Check sheet for the modelled part. Datum: model origin and axes. Units: mm. A direction names the side the tool comes from. Coordinates: 2 decimals unless noted, no trailing zeros. Write each loop counter-clockwise with the first axis right and the second up, starting at its lowest first coordinate (ties: lowest second). Pieces come first, ordered by that corner, then holes. Notation, with made-up numbers: (82, 46.5) - (131, 46.5) arc R24 cw to (131, 72.5) - close; hole circle Ø4 at (61.25, 86). An arc over 180 degrees is marked (long way). Use one line per item in the form item = value. Start each with the question number.
1. Cross-section at B-B on y = 36.5. Record the boundary of the cut face in (x, z).
2. Cross-section at A-A on z = 5.25. Give the number of separate pieces and of enclosed holes in the cut face, then the cut area to 3 significant figures.
3. Scan lines: line 1 along Y through (x, z) = (9.5, 5.5); line 2 along Z through (x, y) = (-29, 30); line 3 along Y through (x, z) = (0, 6.75). Record each from-to range of solid material in increasing order.
4. Draft check along X on faces 1 (the face through (-33.92, 88.5, 6.9)), 2 (the face through (31, 45, 9)), 3 (the face through (-19, 45, 9)), 4 (the face through (13, 55, 14)). Enter one of: +X half, -X half, draft (parallel to the pull), parting line (faces both ways), or undercut.
5. Go/stop test with flat-tipped pins: pin 1 Ø3 at (y, z) = (7.5, 9.5) entering from -X; pin 2 Ø24 at (x, y) = (1, 66) entering from -Z; pin 3 Ø2 at (x, z) = (52.5, 4.5) entering from +Y; pin 4 Ø4 at (x, z) = (42, 11.5) entering from +Y. Record where each tip stops, or that it passes through.
6. Tool access check on faces 5 (the face through (27.92, 47.55, 4.44)), 6 (the face through (6.2, 15, 6.9)), 7 (the face through (59.499, 37, 7)). Record the directions out of +Z, -Z, +X, -X, +Y, -Y that give a thin tool (end or side, any length) a straight path to the whole face; none if there is none.
Autodesk Inventor part; units mm, degrees
ref_plane "YZ Plane" through (0, 0, 0) normal (1, 0, 0) x (0, 1, 0)
ref_plane "XZ Plane" through (0, 0, 0) normal (0, 1, 0) x (-1, 0, 0)
ref_plane "XY Plane" through (0, 0, 0) normal (0, 0, 1) x (1, 0, 0)
sketch "Sketch1" plane through (0, 0, 0) normal (0, 0, 1) x (1, 0, 0)
  line L0 (11.0906, 0.1113) -> (11.0906, 10.1113)
  line L1 (11.0906, 10.1113) -> (1.0906, 20.1113)
  line L2 (31.0918, 20.1126) -> (21.0906, 10.1113)
  line L3 (21.0906, 10.1113) -> (21.0906, 0.1113)
  line L4 (21.0906, 0.1113) -> (11.0906, 0.1113)
  circle A0 centre (16.0906, 16.0413) radius 3.9
  line L5 (37.1863, 89.9817) -> (4.7287, 98.6787)
  line L6 (41.216, 88.9019) -> (37.1863, 89.9817)
  circle A1 centre (31.0906, 45.1113) radius 4
  circle A2 centre (-18.9094, 45.1113) radius 4
  line L7 (1.0906, 20.1113) -> (-38.9094, 20.1113)
  line L8 (4.7287, 98.6787) -> (-28.7852, 107.6587)
  circle A3 centre (6.0906, 62.1113) radius 9
  line L9 (-38.9094, 69.8746) -> (-28.7852, 107.6587)
  line L10 (31.0918, 20.1126) -> (59.4992, 20.1126)
  line L11 (59.4992, 20.1126) -> (59.4992, 54.8735)
  line L12 (59.4992, 84.003) -> (41.216, 88.9019)
  line L13 (59.4992, 54.8735) -> (66.7815, 82.0517)
  line L14 (66.7815, 82.0517) -> (59.4992, 84.003)
  circle A4 centre (48.4066, 52.1126) radius 3.9
  line L15 (-38.9094, 69.8746) -> (-38.9094, 20.1113)
  point P0 (0, 0)
  dimension "d2" = 10
  dimension "d5" = 135
  dimension "d6" = 135
  dimension "d7" = 10
  dimension "d8" = 10
  dimension "d11" = 7.8
  dimension "d14" = 8
  dimension "d15" = 8
  dimension "d16" = 50
  dimension "d20" = 18
  dimension "d21" = 17
  dimension "d24" = 25
  dimension "d30" = 90
  dimension "d31" = 39.117
  dimension "d51" = 7.8
  dimension "d52" = 10
  dimension "d53" = 32
  dimension "d71" = 34.7609
  dimension "d72" = 25
  dimension "d73" = 25
  dimension "d74" = 5
  dimension "d75" = 49.7632
  dimension "d77" = 28.4086
extrude "Extrusion6" add sketch "Sketch1" along normal blind 14
sketch "Sketch6" plane through (59.4992, 20.1126, 0) normal (1, 0, 0) x (0, 0, -1)
  circle A0 centre (-7, 10.2998) radius 3.8217
  line L0 (0, -20.0012) -> (-14, -20.0012)
  point P0 (0, -20.1126)
  dimension "d76" = 30.301
extrude "Extrusion7" cut sketch "Sketch6" against normal blind 120
sketch "Sketch7" plane through (66.7815, 82.0517, 14) normal (0.9659, -0.2588, 0) x (0, 0, -1)
  line L0 (14, 0) -> (0, 0)
  circle A0 centre (7, -10) radius 3.9
  point P0 (14, -96.5401)
  dimension "d58" = 7.8
  dimension "d60" = 10
extrude "Extrusion8" cut sketch "Sketch7" against normal blind 120
sketch "Sketch8" plane through (0, 0, 0) normal (0, 0, -1) x (-1, 0, 0)
  circle A0 centre (-6.0906, 62.1113) radius 9
  circle A1 centre (-6.0906, 62.1113) radius 11
  point P0 (0, 0)
  dimension "d63" = 22
extrude "Extrusion9" cut sketch "Sketch8" against normal blind 7
sketch "Sketch9" plane through (0, 0, 14) normal (0, 0, 1) x (1, 0, 0)
  circle A0 centre (-18.9094, 45.1113) radius 4
  circle A1 centre (31.0906, 45.1113) radius 4
  point P0 (0, 0)
extrude "Extrusion10" add sketch "Sketch9" against normal blind 5
properties part number "Vertex Bottom tensioner left"
Final values:
q1.outline = (-38.91, 0) - (59.5, 0) - (59.5, 14) - (-38.91, 14) - close
q2.separate_pieces = 3
q2.enclosed_holes = 5
q2.area = 5,850 mm²
q3.line_1 = 11.7 to 26.9, 33.93 to 51.65, 72.57 to 83.32, 90.77 to 97.4
q3.line_2 = 0 to 3.2, 10.8 to 14
q3.line_3 = 20.11 to 26.6, 34.23 to 52.95, 71.27 to 85.56, 93.62 to 99.95
q4.face_1 = -X half
q4.face_2 = undercut
q4.face_3 = undercut
q4.face_4 = draft
q5.pin_1 = 11.09
q5.pin_2 = 0
q5.pin_3 = 86.15
q5.pin_4 = 89.23
q6.face_5 = -Z
q6.face_6 = +Z, -Z, -X, -Y
q6.face_7 = +Z, -Z, +X, -Y
